Design review of the part shown in the three views and the two pictorial views. Dimensions are in mm from the part's minimum x, y and z. Round coordinates to 2 decimals unless told otherwise and drop trailing zeros. Write each loop counter-clockwise with the first axis right and the second up, starting at its lowest first coordinate (ties: lowest second). Pieces come first, ordered by that corner, then holes. Notation, with made-up numbers: (20.5, 56.25) -> (77.5, 56.25) arc R25 cw to (77.5, 76.25) -> close; hole circle Ø8 at (22.5, 28). An arc over 180 degrees is marked (long way). One line per question, with ' | ' between items. Start each with the question number.
1) For probe 1 along Y at (x, z) = (176.5, 5); probe 2 along X at (y, z) = (107, 3.5) (1 decimal); probe 3 along Y at (x, z) = (155, 3.5), list the stretches that pass through material, from the lowest coordinate up.
2) Consider section C-C (x = 133). Give the boundary of the cut face in (y, z).
3) Consider section A-A (y = 152.4). Give the boundary of the cut face in (x, z).
4) Consider section B-B (z = 2.5). Give the boundary of the cut face in (x, y).
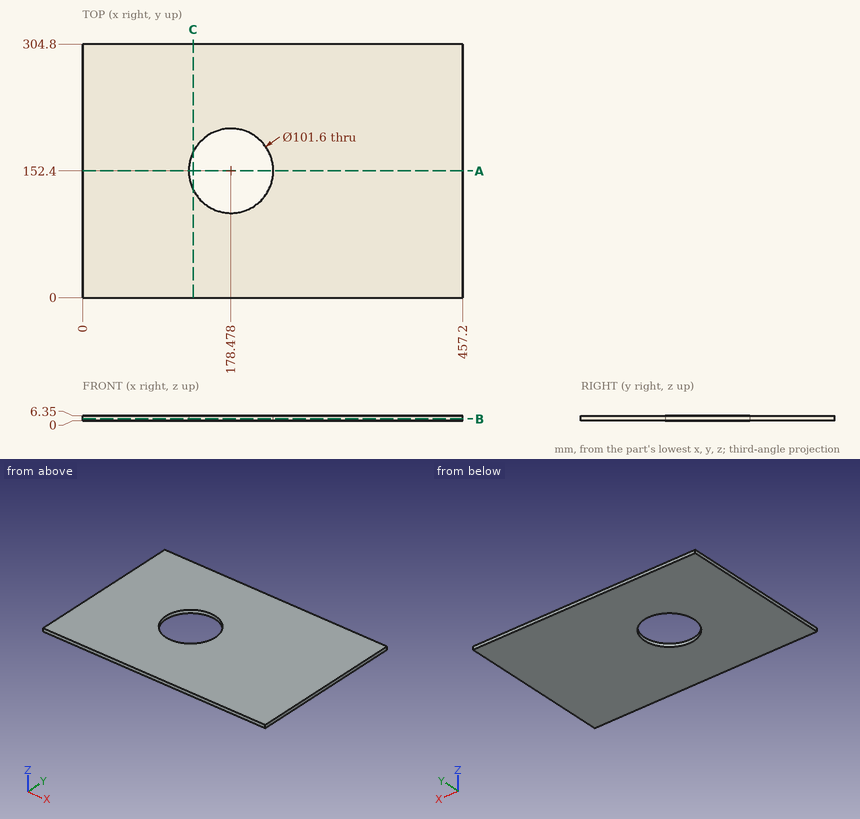
From the geometry:
1) probe 1: y = 0 to 101.64, 203.16 to 304.8 | probe 2: x = 0 to 155.7, 201.3 to 457.2 | probe 3: y = 0 to 107.35, 197.45 to 304.8
2) outline: (0, 0) -> (129.76, 0) -> (129.76, 6.35) -> (0, 6.35) -> close; (175.04, 0) -> (304.8, 0) -> (304.8, 6.35) -> (175.04, 6.35) -> close
3) outline: (0, 0) -> (127.68, 0) -> (127.68, 6.35) -> (0, 6.35) -> close; (229.28, 0) -> (457.2, 0) -> (457.2, 6.35) -> (229.28, 6.35) -> close
4) outline: (0, 0) -> (457.2, 0) -> (457.2, 304.8) -> (0, 304.8) -> close; hole circle Ø101.6 at (178.48, 152.4)
